```python
from build123d import *

# Parameters (mm, degrees)
SKETCH1_R           = 10.72611465
SKETCH1_R_2         = 3.05
BOSS_EXTRUDE1_DEPTH = 6
BOSS_EXTRUDE2_DEPTH = 6


with BuildPart() as part:
    # Sketch1 → Boss-Extrude1 (new body)
    with BuildSketch(Plane.XY):
        Circle(SKETCH1_R)
        Circle(SKETCH1_R_2, mode=Mode.SUBTRACT)
    extrude(amount=BOSS_EXTRUDE1_DEPTH)

    # Sketch3 → Boss-Extrude2 (add)
    with BuildSketch(Plane.XY.offset(6)):
        with BuildLine():
            Line((-13.72611465, 0.5), (-13.72611465, -0.5))
            Line((-13.72611465, -0.5), (-10.620597641, -1.500813525))
            ThreePointArc((-10.620597641, -1.500813525), (-10.72611465, 0), (-10.620597641, 1.500813525))
            Line((-10.620597641, 1.500813525), (-13.72611465, 0.5))
        make_face()
        with BuildLine():
            Line((-12.872618102, 4.790816901), (-10.386489254, 2.677755861))
            ThreePointArc((-10.386489254, 2.677755861), (-9.909637788, 4.10470637), (-9.237816312, 5.450897656))
            Line((-9.237816312, 5.450897656), (-12.48993467, 5.714696433))
            Line((-12.48993467, 5.714696433), (-12.872618102, 4.790816901))
        make_face()
        with BuildLine():
            ThreePointArc((-9.237816312, -5.450897656), (-9.909637788, -4.10470637), (-10.386489254, -2.677755861))
            Line((-10.386489254, -2.677755861), (-12.872618102, -4.790816901))
            Line((-12.872618102, -4.790816901), (-12.48993467, -5.714696433))
            Line((-12.48993467, -5.714696433), (-9.237816312, -5.450897656))
        make_face()
        with BuildLine():
            Line((-10.059382139, 9.352275358), (-8.571132033, 6.448661191))
            ThreePointArc((-8.571132033, 6.448661191), (-7.584508405, 7.584508405), (-6.448661191, 8.571132033))
            Line((-6.448661191, 8.571132033), (-9.352275358, 10.059382139))
            Line((-9.352275358, 10.059382139), (-10.059382139, 9.352275358))
        make_face()
        with BuildLine():
            ThreePointArc((-6.448661191, -8.571132033), (-7.584508405, -7.584508405), (-8.571132033, -6.448661191))
            Line((-8.571132033, -6.448661191), (-10.059382139, -9.352275358))
            Line((-10.059382139, -9.352275358), (-9.352275358, -10.059382139))
            Line((-9.352275358, -10.059382139), (-6.448661191, -8.571132033))
        make_face()
        with BuildLine():
            Line((-5.714696433, 12.48993467), (-5.450897656, 9.237816312))
            ThreePointArc((-5.450897656, 9.237816312), (-4.10470637, 9.909637788), (-2.677755861, 10.386489254))
            Line((-2.677755861, 10.386489254), (-4.790816901, 12.872618102))
            Line((-4.790816901, 12.872618102), (-5.714696433, 12.48993467))
        make_face()
        with BuildLine():
            ThreePointArc((-2.677755861, -10.386489254), (-4.10470637, -9.909637788), (-5.450897656, -9.237816312))
            Line((-5.450897656, -9.237816312), (-5.714696433, -12.48993467))
            Line((-5.714696433, -12.48993467), (-4.790816901, -12.872618102))
            Line((-4.790816901, -12.872618102), (-2.677755861, -10.386489254))
        make_face()
        with BuildLine():
            Line((-0.5, 13.72611465), (-1.500813525, 10.620597641))
            ThreePointArc((-1.500813525, 10.620597641), (0, 10.72611465), (1.500813525, 10.620597641))
            Line((1.500813525, 10.620597641), (0.5, 13.72611465))
            Line((0.5, 13.72611465), (-0.5, 13.72611465))
        make_face()
        with BuildLine():
            ThreePointArc((1.500813525, -10.620597641), (0, -10.72611465), (-1.500813525, -10.620597641))
            Line((-1.500813525, -10.620597641), (-0.5, -13.72611465))
            Line((-0.5, -13.72611465), (0.5, -13.72611465))
            Line((0.5, -13.72611465), (1.500813525, -10.620597641))
        make_face()
        with BuildLine():
            Line((4.790816901, 12.872618102), (2.677755861, 10.386489254))
            ThreePointArc((2.677755861, 10.386489254), (4.10470637, 9.909637788), (5.450897656, 9.237816312))
            Line((5.450897656, 9.237816312), (5.714696433, 12.48993467))
            Line((5.714696433, 12.48993467), (4.790816901, 12.872618102))
        make_face()
        with BuildLine():
            ThreePointArc((5.450897656, -9.237816312), (4.10470637, -9.909637788), (2.677755861, -10.386489254))
            Line((2.677755861, -10.386489254), (4.790816901, -12.872618102))
            Line((4.790816901, -12.872618102), (5.714696433, -12.48993467))
            Line((5.714696433, -12.48993467), (5.450897656, -9.237816312))
        make_face()
        with BuildLine():
            Line((9.352275358, 10.059382139), (6.448661191, 8.571132033))
            ThreePointArc((6.448661191, 8.571132033), (7.584508405, 7.584508405), (8.571132033, 6.448661191))
            Line((8.571132033, 6.448661191), (10.059382139, 9.352275358))
            Line((10.059382139, 9.352275358), (9.352275358, 10.059382139))
        make_face()
        with BuildLine():
            ThreePointArc((8.571132033, -6.448661191), (7.584508405, -7.584508405), (6.448661191, -8.571132033))
            Line((6.448661191, -8.571132033), (9.352275358, -10.059382139))
            Line((9.352275358, -10.059382139), (10.059382139, -9.352275358))
            Line((10.059382139, -9.352275358), (8.571132033, -6.448661191))
        make_face()
        with BuildLine():
            Line((12.48993467, 5.714696433), (9.237816312, 5.450897656))
            ThreePointArc((9.237816312, 5.450897656), (9.909637788, 4.10470637), (10.386489254, 2.677755861))
            Line((10.386489254, 2.677755861), (12.872618102, 4.790816901))
            Line((12.872618102, 4.790816901), (12.48993467, 5.714696433))
        make_face()
        with BuildLine():
            ThreePointArc((10.386489254, -2.677755861), (9.909637788, -4.10470637), (9.237816312, -5.450897656))
            Line((9.237816312, -5.450897656), (12.48993467, -5.714696433))
            Line((12.48993467, -5.714696433), (12.872618102, -4.790816901))
            Line((12.872618102, -4.790816901), (10.386489254, -2.677755861))
        make_face()
        with BuildLine():
            Line((13.72611465, 0.5), (10.620597641, 1.500813525))
            ThreePointArc((10.620597641, 1.500813525), (10.72611465, 0), (10.620597641, -1.500813525))
            Line((10.620597641, -1.500813525), (13.72611465, -0.5))
            Line((13.72611465, -0.5), (13.72611465, 0.5))
        make_face()
    extrude(amount=-BOSS_EXTRUDE2_DEPTH)


solid = part.part
```
CAD build for the part. Positions are in the model's coordinates, mm. A direction names the side the tool comes from. Round coordinates to 2 decimals unless told otherwise and drop trailing zeros. Loops run counter-clockwise (first coordinate to the right, second up) from the corner with the lowest first, then second, coordinate; pieces in that order, holes last. Notation, with made-up numbers: (73, 49) - (111, 49) arc R28 cw to (111, 68) - close; hole circle Ø6 at (-10, 19). An arc over 180 degrees is marked (long way). Return JSON: item names as keys, results as strings. Group by question number.
Q1. Band-saw the part on D-D on y = -7. Give the cut face in (x, z).
Q2. Two-plate mould, pull along X, no slides. Class faces 1 (the face through (12.68, -5.26, 3.04)), 2 (the face through (-10.84, 5.58, 3.04)), 3 (the face through (0, 13.726, 3)): +X half, -X half, draft (parallel to the pull), parting line (faces both ways), or undercut.
Q3. Drill centre lines: line 1 along Y through (x, z) = (0, 4.6); line 2 along X through (y, z) = (-9.75, 0.5); line 3 along X through (y, z) = (10, 3.2). Where is each one in solid material? Low to high. Write a range as [from, to].
Q4. Band-saw the part on C-C on y = -11.25. Give the cut face in (x, z), plus the area to 3 significant figures.
Q5. Band-saw the part on A-A on x = 0. Give the cut face in (y, z), plus the area to 3 significant figures.
Q6. Flat gauge pins, fed straight in: pin 1 Ø10 at (x, y) = (-10.5, 2) entering from -Z; pin 2 Ø1 at (y, z) = (-4.5, 4) entering from -X. Where does each tip first touch, or does it go through?
Q7. Tool access for faces 4 (the face through (7.88, -9.305, 3.042)), 5 (the face through (5.97, 8.91, 2.96)), 6 (the face through (-10.522, -2.084, 2.958)): list every direction of +Z, -Z, +X, -X, +Y, -Y with a clear straight run to the whole face (end or side of a thin tool).
Solutions:
{
 "1": {"outline": "(-8.85, 0) - (8.85, 0) - (8.85, 6) - (-8.85, 6) - close"},
 "2": {"face 1": "+X half", "face 2": "undercut", "face 3": "draft"},
 "3": {"line 1": "y = [-13.73, -3.05], [3.05, 13.73]", "line 2": "x = [-9.66, -8.75], [-5.49, 5.49], [8.75, 9.66]", "line 3": "x = [-9.41, -9.24], [-5.51, 5.51], [9.24, 9.41]"},
 "4": {"outline": "(-5.61, 0) - (-3.41, 0) - (-3.41, 6) - (-5.61, 6) - close; (-1.3, 0) - (1.3, 0) - (1.3, 6) - (-1.3, 6) - close; (3.41, 0) - (5.61, 0) - (5.61, 6) - (3.41, 6) - close", "area": "42.0 mm^2"},
 "5": {"outline": "(-13.73, 0) - (-3.05, 0) - (-3.05, 6) - (-13.73, 6) - close; (3.05, 0) - (13.73, 0) - (13.73, 6) - (3.05, 6) - close", "area": "128 mm^2"},
 "6": {"pin 1": "stops at z = 0", "pin 2": "stops at x = -12.87"},
 "7": {"face 4": "+Z, -Z, -Y", "face 5": "+Z, -Z", "face 6": "+Z, -Z, -X"}
}
